from build123d import *

# Parameters (mm, degrees)
SKETCH1_W               = 177
SKETCH1_H               = 66.3
BOSS_EXTRUDE1_DEPTH     = 10
CUT_EXTRUDE1_DEPTH      = 120.991628317
CUT_EXTRUDE1_DEPTH_BACK = 7
SKETCH2_W               = 171
SKETCH2_H               = 60.3
SKETCH3_W               = 5
SKETCH3_H               = 66.3
BOSS_EXTRUDE2_DEPTH     = 30
SKETCH4_W               = 147
SKETCH4_H               = 66.3
CUT_EXTRUDE2_DEPTH      = 30
SKETCH5_W               = 8
SKETCH5_H               = 8
SKETCH5_R               = 1.899919422
SKETCH5_R_2             = 1.99416254
BOSS_EXTRUDE3_DEPTH     = 3
SKETCH6_W               = 53.200668984
SKETCH6_H               = 118.475248661
CUT_EXTRUDE3_DEPTH      = 137.93353889


with BuildPart() as part:
    # Sketch1 → Boss-Extrude1 (new body)
    with BuildSketch(Plane(origin=(0, 0, 0), x_dir=(1, 0, 0), z_dir=(0, 1, 0))):
        with Locations((-24.496138181, -5.963471112)):
            Rectangle(SKETCH1_W, SKETCH1_H)
    extrude(amount=BOSS_EXTRUDE1_DEPTH)

    # Sketch2 → Cut-Extrude1 (cut, two sides: drawn at the far end of the back side and taken through both)
    with BuildSketch(Plane(origin=(0, 10, 0), x_dir=(1, 0, 0), z_dir=(0, 1, 0)).offset(-CUT_EXTRUDE1_DEPTH_BACK)):
        with Locations((-24.496138181, -5.963471112)):
            Rectangle(SKETCH2_W, SKETCH2_H)
    extrude(amount=CUT_EXTRUDE1_DEPTH + CUT_EXTRUDE1_DEPTH_BACK, mode=Mode.SUBTRACT)

    # Sketch3 → Boss-Extrude2 (add)
    with BuildSketch(Plane.XZ):
        with Locations((-105.496138181, 5.963471112)):
            Rectangle(SKETCH3_W, SKETCH3_H)
        with Locations((56.503861819, 5.963471112)):
            Rectangle(SKETCH3_W, SKETCH3_H)
    extrude(amount=BOSS_EXTRUDE2_DEPTH)

    # Sketch4 → Cut-Extrude2 (cut)
    with BuildSketch(Plane.XZ):
        with Locations((-24.496138181, 5.963471112)):
            Rectangle(SKETCH4_W, SKETCH4_H)
    extrude(amount=-CUT_EXTRUDE2_DEPTH, mode=Mode.SUBTRACT)


with BuildPart() as cut_extrude2_piece_1:
    # of the separate pieces the step leaves, piece 1, a body of its own (cut_extrude2_pieces)
    add(part.part.solids().sort_by_distance((-97.996138181, 0, 39.113471112))[0])



with BuildPart() as cut_extrude2_piece_2:
    # of the separate pieces the step leaves, piece 2, a body of its own (cut_extrude2_pieces)
    add(part.part.solids().sort_by_distance((64.003861819, 0, 39.113471112))[0])


with BuildPart() as cut_extrude2_piece_1_1:
    add(cut_extrude2_piece_1.part)

    add(cut_extrude2_piece_2.part)  # Boss-Extrude3 merges Cut-Extrude2 piece 2
    # Sketch5 → Boss-Extrude3 (add)
    # profile 1 of 2: a face of its own
    with BuildSketch(Plane.XZ.offset(30)):
        with Locations((-111.996138181, 6.113471112)):
            Rectangle(SKETCH5_W, SKETCH5_H)
        with Locations(Location((-111.976969615, 5.996435965, 0), (0, 0, 270))):
            Circle(SKETCH5_R, mode=Mode.SUBTRACT)
    # profile 2 of 2: a face of its own
    with BuildSketch(Plane.XZ.offset(30)):
        with Locations((63.003861819, 6.113471112)):
            Rectangle(SKETCH5_W, SKETCH5_H)
        with Locations(Location((63.046032676, 6.021165831, 0), (0, 0, 270))):
            Circle(SKETCH5_R_2, mode=Mode.SUBTRACT)
    extrude(amount=-BOSS_EXTRUDE3_DEPTH)

    # Sketch6 → Cut-Extrude3 (cut, through all)
    with BuildSketch(Plane(origin=(0, 0, -27.186528888), x_dir=(-1, 0, 0), z_dir=(0, 0, -1))):
        with Locations((95.157985418, 15.958745635)):
            Rectangle(SKETCH6_W, SKETCH6_H)
    extrude(amount=-CUT_EXTRUDE3_DEPTH, mode=Mode.SUBTRACT)


solid = cut_extrude2_piece_1_1.part
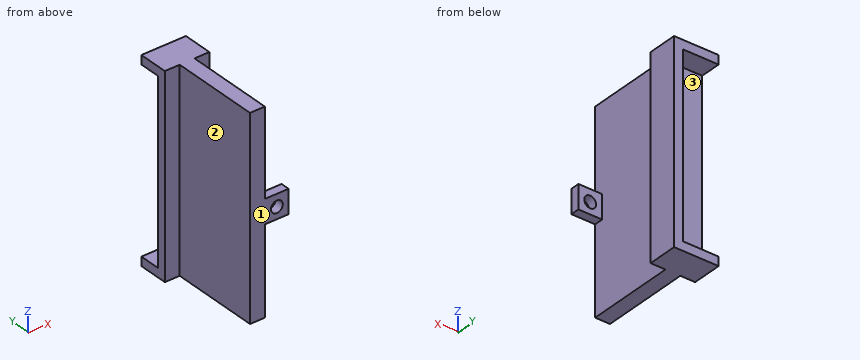
Work out the finished part from the listing and answer in its coordinate system (mm). Face numbers are marked on the shaded views. A direction names the side the tool comes from. Coordinates: 2 decimals unless noted, no trailing zeros. Loops run counter-clockwise (first coordinate to the right, second up) from the corner with the lowest first, then second, coordinate; pieces in that order, holes last. Notation, with made-up numbers: (85.25, 85) -> (112.25, 85) arc R9 cw to (112.25, 90) -> close; hole circle Ø5 at (85.25, -32). An arc over 180 degrees is marked (long way). Answer as CSV lines item,"result".
1) The part is cut by section B-B (x = 60.25). Give the vertices of the cut face in (y, z), and give its area (3 significant figures).
A:
outline,"(-30, 2.11) -> (-27, 2.11) -> (-27, 10.11) -> (-30, 10.11) -> close; (0, -27.19) -> (10, -27.19) -> (10, -24.19) -> (3, -24.19) -> (3, 36.11) -> (10, 36.11) -> (10, 39.11) -> (0, 39.11) -> close"
area,"265 mm²"
2) Flat-ended cylindrical pins translate along their axes: pin 1 (0.9 mm diameter, centred on x = 64, y = -28, fed in from -Z); pin 2 (1 mm diameter, centred on y = 3, z = 4, fed in from +X); pin 3 (8 mm diameter, centred on x = 52.5, z = 25.5, fed in from +Y); pin 4 (10 mm diameter, centred on x = 60.5, z = -13.5, fed in from -Y). Find the tip coordinate at first contact, or state that the pin passes through.
A:
pin 1,"stops at z = 2.11"
pin 2,"stops at x = 64"
pin 3,"stops at y = 3"
pin 4,"stops at y = -30"
3) The part is cut by section C-C (y = 4). Give the vertices of the cut face in (x, z), and give its area (3 significant figures).
A:
outline,"(49, -27.19) -> (64, -27.19) -> (64, 39.11) -> (49, 39.11) -> (49, 36.11) -> (61, 36.11) -> (61, -24.19) -> (49, -24.19) -> close"
area,"271 mm²"
4) The part is cut by section D-D (x = 51.5). Give the vertices of the cut face in (y, z), and give its area (3 significant figures).
A:
outline,"(0, -27.19) -> (10, -27.19) -> (10, -24.19) -> (3, -24.19) -> (3, 36.11) -> (10, 36.11) -> (10, 39.11) -> (0, 39.11) -> close"
area,"241 mm²"
5) Straight lines are drawn through the part: probe 1 along Z at (x, y) = (59.5, 6); probe 2 along Y at (x, z) = (51, -5); probe 3 along Y at (x, z) = (55, 32). For each, find the intervals that lie inside material, in ascending order.
A:
probe 1,"z = -27.19 to -24.19, 36.11 to 39.11"
probe 2,"y = 0 to 3"
probe 3,"y = -30 to 3"
6) For the marked faces 1, 2 and 3, determine the directions among +Z, -Z, +X, -X, +Y, -Y from which every point of the face is accessible in a straight line to the end or side of a thin tool.
A:
face 1,"+Z, -Z, +X, -X, -Y"
face 2,"+Z, -Z, -X, -Y"
face 3,"-X, +Y"
7) The part is cut by section A-A (z = -3). Give the vertices of the cut face in (x, y), and give its area (3 significant figures).
A:
outline,"(49, 0) -> (54, 0) -> (54, -30) -> (59, -30) -> (59, 0) -> (64, 0) -> (64, 10) -> (61, 10) -> (61, 3) -> (49, 3) -> close"
area,"216 mm²"
